Autodesk Inventor part; units mm, degrees
ref_plane "YZ Plane" through (0, 0, 0) normal (1, 0, 0) x (0, 1, 0)
ref_plane "XZ Plane" through (0, 0, 0) normal (0, 1, 0) x (-1, 0, 0)
ref_plane "XY Plane" through (0, 0, 0) normal (0, 0, 1) x (1, 0, 0)
sketch "Эскиз1" plane through (0, 0, 0) normal (0, 0, 1) x (1, 0, 0)
  circle A0 centre (0, 44.0756) radius 40
  point P0 (0, 0)
  dimension "d0" = 80
extrude "Выдавливание1" add sketch "Эскиз1" along normal blind 5
sketch "Эскиз2" plane through (0, 44.0756, 0) normal (0, 0, -1) x (-1, 0, 0)
  line L0 (0, 4) -> (-3.4641, 2)
  line L1 (-3.4641, 2) -> (-3.4641, -2)
  line L2 (-3.4641, -2) -> (0, -4)
  line L3 (0, -4) -> (3.421, -2.0249)
  line L4 (3.421, -2.0249) -> (3.4641, 2)
  line L5 (3.4641, 2) -> (0, 4)
  point P0 (0, -44.0756)
  point P1 (0, 0)
extrude "Выдавливание2" cut sketch "Эскиз2" against normal blind 4
sketch "Эскиз3" plane through (0, 44.0756, 5) normal (0, 0, 1) x (1, 0, 0)
  circle A0 centre (0, 0) radius 40
  circle A1 centre (0, 0) radius 38
  point P0 (0, -44.0756)
  dimension "d5" = 2
extrude "Выдавливание3" add sketch "Эскиз3" along normal blind 5 contours A1
sketch "Эскиз5" plane through (0, 44.0756, 10) normal (0, 0, 1) x (1, 0, 0)
  circle A0 centre (0, 0) radius 38
  point P0 (0, -44.0756)
hole "Отверстие1" at (0, 44.0756, 10) direction (0, 0, -1) diameter 4.5 end through all countersink diameter 8 countersink angle 90
properties part number "Cap-01"
Verification items for the finished model (mm, model axes). A direction names the side the tool comes from. Coordinates: 2 decimals unless noted, no trailing zeros. Loops run counter-clockwise (first coordinate to the right, second up) from the corner with the lowest first, then second, coordinate; pieces in that order, holes last. Notation, with made-up numbers: (57, 59) - (81, 59) arc R25 cw to (81, 90) - close; hole circle Ø4 at (-11, 43). An arc over 180 degrees is marked (long way). Return JSON: item names as keys, results as strings.
1. Section check C-C, the plane y = 24. Record the boundary of the cut face in (x, z).
Established:
{"outline": "(-34.6, 0) - (34.6, 0) - (34.6, 5) - (32.26, 5) - (32.26, 10) - (-32.26, 10) - (-32.26, 5) - (-34.6, 5) - close"}
2. Section check D-D, the plane z = 6.5. Record the boundary of the cut face in (x, y), then the cut area to 3 significant figures.
Established:
{"outline": "circle Ø76 at (0, 44.08); hole circle Ø4.5 at (0, 44.08)", "area": "4,520 mm2"}
3. Section check B-B, the plane x = -21. Record the boundary of the cut face in (y, z), then the cut area to 3 significant figures.
Established:
{"outline": "(10.03, 0) - (78.12, 0) - (78.12, 5) - (75.75, 5) - (75.75, 10) - (12.41, 10) - (12.41, 5) - (10.03, 5) - close", "area": "657 mm2"}
4. Go/stop test with flat-tipped pins: pin 1 (5 mm diameter, centred on x = -29.5, z = 8.5, fed in from +Y); pin 2 (3 mm diameter, centred on y = 61.5, z = 8.5, fed in from +X). Record where each tip stops, or that it passes through.
Established:
{"pin 1": "stops at y = 70.82", "pin 2": "stops at x = 34.5"}
5. Thickness scan on L1, parallel to Y at x = 0, z = 5.25; L2, parallel to X at y = 47, z = 0.75; L3, parallel to X at y = 78, z = 7. Record the ranges inside material, lowest first.
Established:
{"L1": "y = 6.08 to 41.83, 46.33 to 82.08", "L2": "x = -39.89 to -1.86, 1.86 to 39.89", "L3": "x = -17.12 to 17.12"}
6. Mould release check, pull along X, two halves, no side actions. Record for faces 3 (the cylindrical face through (17.53, 77.79, 7.46)), 4 (the flat face through (35.4, 29.4, 5)), 5 (the cylindrical face through (-0.099, 46.323, 6.095)): +X half, -X half, draft (parallel to the pull), parting line (faces both ways), or undercut.
Established:
{"face 3": "parting line", "face 4": "draft", "face 5": "undercut"}
7. Tool access check on faces 1 (the cylindrical face through (-5.207, 4.416, 2.465)), 2 (the flat face through (-1.76, 47.06, 1.97)). Record the directions out of +Z, -Z, +X, -X, +Y, -Y that give a thin tool (end or side, any length) a straight path to the whole face; none if there is none.
Established:
{"face 1": "+Z, -Z", "face 2": "-Z"}
8. Section check A-A, the plane z = 2. Record the boundary of the cut face in (x, y).
Established:
{"outline": "circle Ø80 at (0, 44.08); hole (-3.46, 46.08) - (-3.42, 42.05) - (0, 40.08) - (3.46, 42.08) - (3.46, 46.08) - (0, 48.08) - close"}
